Model file for the job. Use its own axes, mm. A direction names the side the tool comes from. Round coordinates to 2 decimals unless told otherwise and drop trailing zeros. Write each loop counter-clockwise with the first axis right and the second up, starting at its lowest first coordinate (ties: lowest second). Pieces come first, ordered by that corner, then holes. Notation, with made-up numbers: (22, -34) - (58, -34) arc R27 cw to (58, 3) - close; hole circle Ø11 at (39, 16.25). An arc over 180 degrees is marked (long way). One line per item, written item: value.
from build123d import *

# Parameters (mm, degrees)
SKETCH_1_W      = 5.5
SKETCH_1_H      = 5.5
EXTRUDE_1_DEPTH = 5.5


with BuildPart() as part:
    # ｽｹｯﾁ1 → ﾎﾞｽ - 押し出し1 (new body)
    with BuildSketch(Plane.XY):
        Polygon((-6.75, 5), (-6.75, -5), (12.75, -5), (12.75, -46), (22.75, -46), (22.75, 54), (12.75, 54), (12.75, 44), (-6.75, 44), (-6.75, 34), (12.75, 34), (12.75, 5), align=None)
        Rectangle(SKETCH_1_W, SKETCH_1_H, mode=Mode.SUBTRACT)
        with Locations((0, 39)):
            Rectangle(SKETCH_1_W, SKETCH_1_H, mode=Mode.SUBTRACT)
    extrude(amount=EXTRUDE_1_DEPTH)


solid = part.part
1. Band-saw the part on A-A on x = -1.5. Write the cut outline in (y, z), plus the area to 3 significant figures.
Report:
outline: (-5, 0) - (-2.75, 0) - (-2.75, 5.5) - (-5, 5.5) - close; (2.75, 0) - (5, 0) - (5, 5.5) - (2.75, 5.5) - close; (34, 0) - (36.25, 0) - (36.25, 5.5) - (34, 5.5) - close; (41.75, 0) - (44, 0) - (44, 5.5) - (41.75, 5.5) - close
area: 49.5 mm²
2. Band-saw the part on B-B on z = 1. Write the cut outline in (x, y), plus the area to 3 significant figures.
Report:
outline: (-6.75, -5) - (12.75, -5) - (12.75, -46) - (22.75, -46) - (22.75, 54) - (12.75, 54) - (12.75, 44) - (-6.75, 44) - (-6.75, 34) - (12.75, 34) - (12.75, 5) - (-6.75, 5) - close; hole (-2.75, -2.75) - (2.75, -2.75) - (2.75, 2.75) - (-2.75, 2.75) - close; hole (-2.75, 36.25) - (2.75, 36.25) - (2.75, 41.75) - (-2.75, 41.75) - close
area: 1,330 mm²
3. Mould opens along Y. For faces 1 (the face through (0, 41.75, 3)), 2 (the face through (22.75, 3, 3)), 3 (the face through (3, -5, 3)) say: released by +Y, released by -Y, zero draft, split by the parting line, or undercut.
Report:
face 1: undercut
face 2: zero draft
face 3: released by -Y
4. Band-saw the part on C-C on x = 3.75. Write the cut outline in (y, z).
Report:
outline: (-5, 0) - (5, 0) - (5, 5.5) - (-5, 5.5) - close; (34, 0) - (44, 0) - (44, 5.5) - (34, 5.5) - close
5. Tool access for faces 4 (the face through (3, 44, 3)), 5 (the face through (12.75, 20, 3)), 6 (the face through (12.75, -25, 3)), 7 (the face through (0, 2.75, 3)): list every direction of +Z, -Z, +X, -X, +Y, -Y with a clear straight run to the whole face (end or side of a thin tool).
Report:
face 4: +Z, -Z, -X, +Y
face 5: +Z, -Z, -X
face 6: +Z, -Z, -X, -Y
face 7: +Z, -Z
6. Wall check: probe 1 along Y at (x, z) = (-2, 4.7); probe 2 along Y at (x, z) = (12, 3.8); probe 3 along X at (y, z) = (-20, 3.1). Give the ranges that are in metal, low to high. Write a range as [from, to].
Report:
probe 1: [-5, -2.75], [2.75, 5], [34, 36.25], [41.75, 44]
probe 2: [-5, 5], [34, 44]
probe 3: [12.75, 22.75]
7. Band-saw the part on D-D on y = -33.5. Write the cut outline in (x, z), plus the area to 3 significant figures.
Report:
outline: (12.75, 0) - (22.75, 0) - (22.75, 5.5) - (12.75, 5.5) - close
area: 55.0 mm²
8. Drop flat-ended pins along their axis: pin 1 (1.5 mm diameter, centred on x = 4.5, z = 1, fed in from +Y); pin 2 (1.6 mm diameter, centred on x = 7.5, z = 4, fed in from -Y); pin 3 (3 mm diameter, centred on y = 28, z = 1.5, fed in from -X); pin 4 (8 mm diameter, centred on x = 3.5, y = -10, fed in from -Z). Give the stop position or say it passes through.
Report:
pin 1: y = 44
pin 2: y = -5
pin 3: x = 12.75
pin 4: through
